```python
from build123d import *

# Parameters (mm, degrees)
SKETCH1_R           = 17.5
SKETCH1_R_2         = 15
BOSS_EXTRUDE1_DEPTH = 30


with BuildPart() as part:
    # Sketch1 → Boss-Extrude1 (new body)
    with BuildSketch(Plane(origin=(0, 0, 0), x_dir=(0, 0, -1), z_dir=(1, 0, 0))):
        with BuildLine():
            Line((0, 249.289321881), (0, 20))
            ThreePointArc((0, 20), (5.857864376, 5.857864376), (20, 0))
            Line((20, 0), (456.16, 0))
            Line((456.16, 0), (892.32, 0))
            ThreePointArc((892.32, 0), (906.462135624, 5.857864376), (912.32, 20))
            Line((912.32, 20), (912.32, 258.272384904))
            ThreePointArc((912.32, 258.272384904), (908.177363781, 278.199807895), (896.435912518, 294.825148317))
            Line((896.435912518, 294.825148317), (776.727753487, 406.552763412))
            ThreePointArc((776.727753487, 406.552763412), (760.947077938, 416.516868825), (742.611840969, 420))
            Line((742.611840969, 420), (170.710678119, 420))
            ThreePointArc((170.710678119, 420), (151.5765065, 416.193976626), (135.355339059, 405.355339059))
            Line((135.355339059, 405.355339059), (14.644660941, 284.644660941))
            ThreePointArc((14.644660941, 284.644660941), (3.806023374, 268.4234935), (0, 249.289321881))
        make_face()
        with Locations((40, 32.245311268)):
            Circle(SKETCH1_R, mode=Mode.SUBTRACT)
        with Locations((872.32, 223.507722896)):
            Circle(SKETCH1_R, mode=Mode.SUBTRACT)
        with Locations((872.32, 32.245311268)):
            Circle(SKETCH1_R, mode=Mode.SUBTRACT)
        with Locations((606.16, 162.057722896)):
            Circle(SKETCH1_R, mode=Mode.SUBTRACT)
        with Locations((306.16, 162.057722896)):
            Circle(SKETCH1_R, mode=Mode.SUBTRACT)
        with BuildLine():
            ThreePointArc((456.16, 177.057722896), (471.16, 162.057722896), (456.16, 147.057722896))
            ThreePointArc((456.16, 147.057722896), (441.16, 162.057722896), (456.16, 177.057722896))
        make_face(mode=Mode.SUBTRACT)
        with Locations((40, 223.507722896)):
            Circle(SKETCH1_R_2, mode=Mode.SUBTRACT)
    extrude(amount=BOSS_EXTRUDE1_DEPTH)


solid = part.part
```
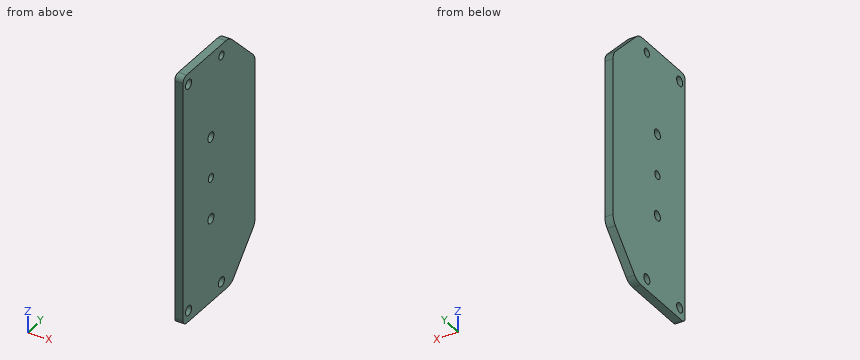
Design review of the part built by this model. Coordinates are the model's own, in mm. Give positions to 0.01 mm unless a question says otherwise; leave off trailing zeros. Loops run counter-clockwise (first coordinate to the right, second up) from the corner with the lowest first, then second, coordinate; pieces in that order, holes last. Notation, with made-up numbers: M -3.5,64.25 L 9.5,64.25 A28 ccw 9.5,82.25 Z; hole C -28.75,29 d10. An arc over 180 degrees is marked long. Return JSON: item names as keys, results as strings. Group by question number.
Item 1: Insertion check: pin 1 Ø21 at (y, z) = (162.06, -306.16) entering from -X; pin 2 Ø1 at (x, y) = (17.5, 279) entering from -Z; pin 3 Ø3 at (x, y) = (5.5, 360.5) entering from -Z; pin 4 Ø6 at (x, z) = (25.5, -132) entering from +Y. Each pin has a flat end and moves straight along its axis. Give the tip position at first contact, or say it passes through.
Item 2: We need section D-D (z = -306.16). Give the boundary of the cut face in (x, y), and give its area (4 significant figures).
Item 3: For probe 1 along Y at (x, z) = (25, -869); probe 2 along Z at (x, y) = (27, 23); probe 3 along Y at (x, z) = (13.75, -606.16), list the stretches that pass through material, from the lowest coordinate up.
Item 4: We need section A-A (z = -456.16). Give the boundary of the cut face in (x, y).
Item 5: We need section B-B (z = -40). Give the boundary of the cut face in (x, y), and give its area (3 significant figures).
Item 6: We need section C-C (x = 24.75). Give the boundary of the cut face in (y, z).
Output:
{
 "1": {"pin 1": "passes through", "pin 2": "stops at z = -908.05", "pin 3": "stops at z = -827.68", "pin 4": "stops at y = 405"},
 "2": {"outline": "M 0,0 L 30,0 L 30,144.56 L 0,144.56 Z; M 0,179.56 L 30,179.56 L 30,420 L 0,420 Z", "area": "11,550 mm^2"},
 "3": {"probe 1": "y = 0 to 15.06, 49.43 to 206.33, 240.69 to 320.43", "probe 2": "z = -912.32 to -887.18, -857.46 to -54.86, -25.14 to 0", "probe 3": "y = 0 to 144.56, 179.56 to 420"},
 "4": {"outline": "M 0,0 L 30,0 L 30,147.06 L 0,147.06 Z; M 0,177.06 L 30,177.06 L 30,420 L 0,420 Z"},
 "5": {"outline": "M 0,0 L 30,0 L 30,14.75 L 0,14.75 Z; M 0,49.75 L 30,49.75 L 30,208.51 L 0,208.51 Z; M 0,238.51 L 30,238.51 L 30,310 L 0,310 Z", "area": "7,350 mm^2"},
 "6": {"outline": "M 0,-892.32 A20 ccw 20,-912.32 L 258.27,-912.32 A50 ccw 294.83,-896.44 L 406.55,-776.73 A50 ccw 420,-742.61 L 420,-170.71 A50 ccw 405.36,-135.36 L 284.64,-14.64 A50 ccw 249.29,0 L 20,0 A20 ccw 0,-20 Z; hole C 32.25,-872.32 d35; hole C 32.25,-40 d35; hole C 162.06,-606.16 d35; hole C 162.06,-306.16 d35; hole C 162.06,-456.16 d30; hole C 223.51,-872.32 d35; hole C 223.51,-40 d30"}
}
